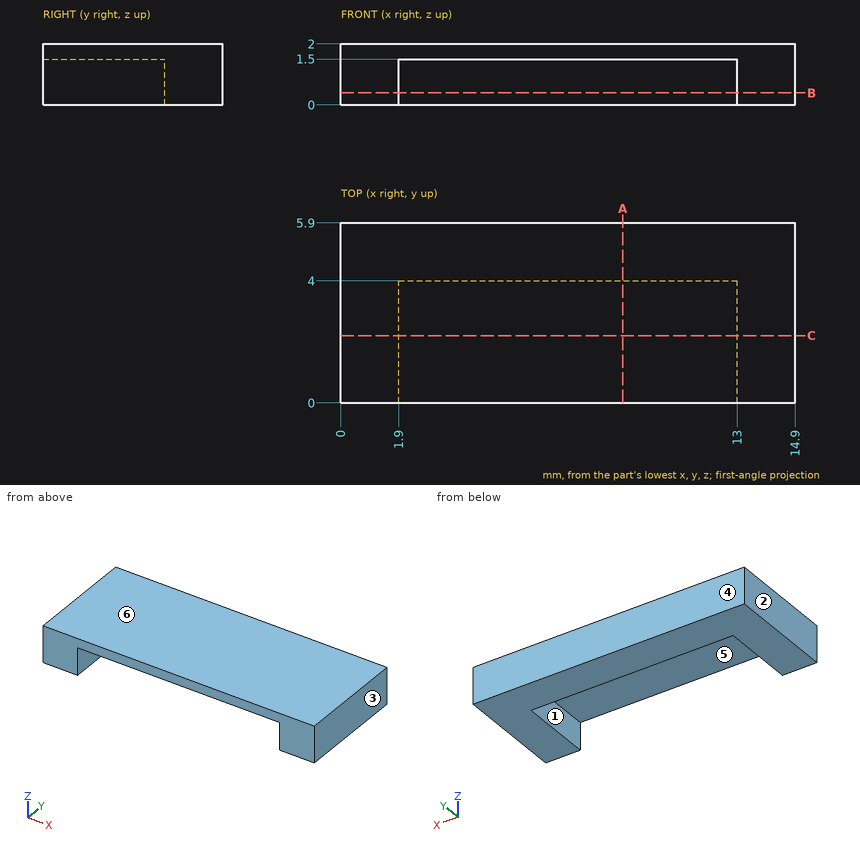
Design review of the part shown in the three views and the two pictorial views. Dimensions are in mm from the part's minimum x, y and z. A direction names the side the tool comes from. Round coordinates to 2 decimals unless told otherwise and drop trailing zeros. Write each loop counter-clockwise with the first axis right and the second up, starting at its lowest first coordinate (ties: lowest second). Pieces come first, ordered by that corner, then holes. Notation, with made-up numbers: (53, 5) - (112, 5) arc R29 cw to (112, 40) - close; hole circle Ø3 at (63.25, 0.5). An arc over 180 degrees is marked (long way). Return JSON: item names as keys, results as strings. Group by question number.
Item 1: We need section C-C on y = 2.2. Write out the cut boundary in (x, z).
Item 2: Machinability: for the marked faces 5 and 6, which of the approach directions +Z, -Z, +X, -X, +Y, -Y give a long, thin tool a straight path to every point of the face, cutting with its end or side? Answer none if there is none.
Item 3: We need section B-B on z = 0.4. Write out the cut boundary in (x, y), and give its area (3 significant figures).
Item 4: We need section A-A on x = 9.25. Write out the cut boundary in (y, z), and give its area (3 significant figures).
Item 5: For probe 1 along X at (y, z) = (0.65, 0.55); probe 2 along Z at (x, y) = (7.75, 2.3); probe 3 along Y at (x, z) = (4.25, 1.15), list the stretches that pass through material, from the lowest coordinate up. Write a range as [from, to].
Item 6: The part is to be moulded in two halves that separate along X. For the marked faces 1, 2, 3 and 4, say which applies: pulls with the +X half, pulls with the -X half, needs draft (parallel to the pull), parting line crosses it, or undercut.
Item 7: Insertion check: P1, Ø2, axis at x = 3.5, y = 4, coming from the -Z side; P2, Ø0.8, axis at x = 7, z = 0.5, coming from the -Y side; P3, Ø1.2, axis at x = 5.5, y = 1.5, coming from the -Z side. Each pin has a flat end and moves straight along its axis. Give the tip position at first contact, or say it passes through.
Model answer:
{
 "1": {"outline": "(0, 0) - (1.9, 0) - (1.9, 1.5) - (13, 1.5) - (13, 0) - (14.9, 0) - (14.9, 2) - (0, 2) - close"},
 "2": {"face 5": "-Z, -Y", "face 6": "+Z, +X, -X, +Y, -Y"},
 "3": {"outline": "(0, 0) - (1.9, 0) - (1.9, 4) - (13, 4) - (13, 0) - (14.9, 0) - (14.9, 5.9) - (0, 5.9) - close", "area": "43.5 mm²"},
 "4": {"outline": "(0, 1.5) - (4, 1.5) - (4, 0) - (5.9, 0) - (5.9, 2) - (0, 2) - close", "area": "5.80 mm²"},
 "5": {"probe 1": "x = [0, 1.9], [13, 14.9]", "probe 2": "z = [1.5, 2]", "probe 3": "y = [4, 5.9]"},
 "6": {"face 1": "undercut", "face 2": "pulls with the -X half", "face 3": "pulls with the +X half", "face 4": "needs draft"},
 "7": {"P1": "stops at z = 0", "P2": "stops at y = 4", "P3": "stops at z = 1.5"}
}
